Source: CAD feature listing. Evaluate the final solid. Frame: model axes, mm. Round coordinates to 2 decimals unless told otherwise and drop trailing zeros. Loops run counter-clockwise (first coordinate to the right, second up) from the corner with the lowest first, then second, coordinate; pieces in that order, holes last. Notation, with made-up numbers: M -7,24 L 26,24 A36 cw 26,63 Z; hole C 50.5,42 d7. An arc over 180 degrees is marked long. Answer as a JSON object with one key per item and string values.
from build123d import *

# Parameters (mm, degrees)
CROQUIS1_R                 = 32.5
CROQUIS1_R_2               = 30
SALIENTE_EXTRUIR1_DEPTH    = 250
CORTAR_EXTRUIR1_REACH      = 256.19
CORTAR_EXTRUIR1_END_RADIUS = 32.5
CROQUIS2_W                 = 5
CROQUIS2_H                 = 20


with BuildPart() as part:
    # Croquis1 → Saliente-Extruir1 (new, symmetric)
    with BuildSketch(Plane(origin=(0, 0, 0), x_dir=(1, 0, 0), z_dir=(0, 1, 0))):
        with Locations(Location((0, 0, 0), (0, 0, 270))):
            Circle(CROQUIS1_R)
        with Locations(Location((0, 0, 0), (0, 0, 270))):
            Circle(CROQUIS1_R_2, mode=Mode.SUBTRACT)
    extrude(amount=SALIENTE_EXTRUIR1_DEPTH, both=True)

    # Cortar-Extruir1: up to this cylinder (the profile starts inside it)
    cortar_extruir1_end = Plane(origin=(0, 0, 0), z_dir=(0, -1, 0)) * Cylinder(CORTAR_EXTRUIR1_END_RADIUS, 1058.38, mode=Mode.PRIVATE)
    # Croquis2 → Cortar-Extruir1 (cut, up to the surface)
    with BuildSketch(Plane.XY, mode=Mode.PRIVATE) as cortar_extruir1_sk1:
        with Locations((0, -240)):
            Rectangle(CROQUIS2_W, CROQUIS2_H)
    cortar_extruir1_tool1 = extrude(cortar_extruir1_sk1.sketch, amount=-CORTAR_EXTRUIR1_REACH, mode=Mode.PRIVATE) & cortar_extruir1_end
    add(cortar_extruir1_tool1.solids().sort_by_distance((0, -240, 0))[0], mode=Mode.SUBTRACT)
    # Croquis2 → Cortar-Extruir1 (cut, up to the surface)
    with BuildSketch(Plane.XY, mode=Mode.PRIVATE) as cortar_extruir1_sk2:
        with Locations((0, 240)):
            Rectangle(CROQUIS2_W, CROQUIS2_H)
    cortar_extruir1_tool2 = extrude(cortar_extruir1_sk2.sketch, amount=-CORTAR_EXTRUIR1_REACH, mode=Mode.PRIVATE) & cortar_extruir1_end
    add(cortar_extruir1_tool2.solids().sort_by_distance((0, 240, 0))[0], mode=Mode.SUBTRACT)


solid = part.part
Item 1: Line query: probe 1 along X at (y, z) = (82.5, 0); probe 2 along Z at (x, y) = (-22, -148); probe 3 along Z at (x, y) = (24, -60.5). Output: solid intervals per line, ascending. Write a range as from..to.
Answer sheet:
{"probe 1": "x = -32.5..-30, 30..32.5", "probe 2": "z = -23.92..-20.4, 20.4..23.92", "probe 3": "z = -21.91..-18, 18..21.91"}
Item 2: Contact query for flat-ended pins moving along their axis: pin 1 Ø10 at (y, z) = (-174, 22) entering from +X; pin 2 Ø2 at (x, y) = (24.5, -150) entering from +Z; pin 3 Ø6 at (y, z) = (194, 18) entering from +X. Output: stop coordinate, or through.
Answer sheet:
{"pin 1": "stops at x = 27.7", "pin 2": "stops at z = 22.45", "pin 3": "stops at x = 28.83"}
Item 3: Pull-direction query (X, two-part tool) for faces 1 (the flat face through (-9, -250, 29)), 2 (the cylindrical face through (9.76, 3.5, 31)), 3 (the cylindrical face through (1.32, -3.5, -29.97)); classes: pulls with the +X half, pulls with the -X half, needs draft (parallel to the pull), parting line crosses it, or undercut.
Answer sheet:
{"face 1": "needs draft", "face 2": "parting line crosses it", "face 3": "undercut"}
Item 4: Section A-A on z = 0. Return the cut outline in (x, y), then the cut area to 3 significant figures.
Answer sheet:
{"outline": "M -32.5,-250 L -30,-250 L -30,250 L -32.5,250 Z; M 30,-250 L 32.5,-250 L 32.5,250 L 30,250 Z", "area": "2,500 mm²"}
Item 5: Section C-C on y = 16. Return the cut outline in (x, z), then the cut area to 3 significant figures.
Answer sheet:
{"outline": "C 0,0 d65; hole C 0,0 d60", "area": "491 mm²"}
Item 6: Section B-B on x = -14. Return the cut outline in (y, z), then the cut area to 3 significant figures.
Answer sheet:
{"outline": "M -250,-29.33 L 250,-29.33 L 250,-26.53 L -250,-26.53 Z; M -250,26.53 L 250,26.53 L 250,29.33 L -250,29.33 Z", "area": "2,800 mm²"}
